Geometry: final body of the model. Coordinates: model frame, mm. A direction names the side the tool comes from. Round coordinates to 2 decimals unless told otherwise and drop trailing zeros. Order: outer loops, then holes, each group sorted by start corner. A loop starts at its lowest first (then second) coordinate and runs counter-clockwise, first axis right, second up. Notation, with made-up numbers: M -22.5,82 L 31.5,82 A29 ccw 31.5,106 Z; hole C -33.5,42 d10. An arc over 180 degrees is marked long. Put each result on its own line as item: value. Start each with the question number.
1) Material intervals for probe 1 along Z at (x, y) = (55, -3); probe 2 along X at (y, z) = (-4, 17.5); probe 3 along Y at (x, z) = (-53.5, 21), sorted ascending. Write a range as [from, to].
2) Section A-A, the plane x = -55. Return loops of the section in (y, z), then the cut area to 3 significant figures.
3) Section B-B, the plane z = 23. Return loops of the section in (x, y).
4) Section C-C, the plane y = -35. Return loops of the section in (x, z).
5) Section D-D, the plane y = -6.5. Return loops of the section in (x, z), then the cut area to 3 significant figures.
6) First-contact query: P1, Ø15, axis at y = -42.5, z = 20, coming from the -X side; P2, Ø2, axis at x = -16.5, y = -29.5, coming from the -Z side; P3, Ø1.5, axis at y = -59.5, z = 17.5, coming from the +X side; P4, Ø12, axis at x = 32, y = -71, coming from the +Z side. Flat tips, straight axial feed; report the tip coordinate or a pass-through.
7) Draft query along Y for faces 1 (the flat face through (-59, -15, 19)), 2 (the cylindrical face through (-59, -8, 12)), 3 (the cylindrical face through (1, -35, -10)). Return one class per face: pulls with the +Y half, pulls with the -Y half, needs draft (parallel to the pull), parting line crosses it, or undercut.
8) Access query for faces 4 (the flat face through (-55, -43, 0)), 5 (the flat face through (55, -43, 0)), 6 (the cylindrical face through (0, -75, 15)). Directions: +Z, -Z, +X, -X, +Y, -Y. A direction counts if a zero-diameter tool reaches every point of the face in a straight line with its end or side. Return the directions, or none.
from build123d import *

# Parameters (mm, degrees)
F0_W      = 140
F0_H      = 60
F1_DEPTH  = 70
F3_DEPTH  = 165
F4_W      = 30
F4_H      = 30
F5_DEPTH  = 55
F6_W      = 30
F6_H      = 30
F7_DEPTH  = 55
F8_R      = 5
F9_DEPTH  = 40
F10_R     = 5
F11_DEPTH = 40
F13_DEPTH = 100
F14_DEPTH = 10


with BuildPart() as f1:
    # F0 (on Front) → F1 (new body)
    with BuildSketch(Plane.XZ):
        Rectangle(F0_W, F0_H)
    extrude(amount=F1_DEPTH)

    # F2 (on face) → F3 (cut, symmetric)
    with BuildSketch(Plane.YZ.offset(70)):
        with BuildLine():
            Line((-55, -30), (-15, -30))
            ThreePointArc((-15, -30), (-35, -10), (-55, -30))
        make_face()
    extrude(amount=F3_DEPTH, both=True, mode=Mode.SUBTRACT)

    # F4 (on face) → F5 (cut)
    with BuildSketch(Plane.XZ.offset(70)):
        with Locations((55, 15)):
            Rectangle(F4_W, F4_H)
    extrude(amount=-F5_DEPTH, mode=Mode.SUBTRACT)

    # F6 (on face) → F7 (cut)
    with BuildSketch(Plane.XZ.offset(70)):
        with Locations((-55, 15)):
            Rectangle(F6_W, F6_H)
    extrude(amount=-F7_DEPTH, mode=Mode.SUBTRACT)

    # F8 (on face) → F9 (cut)
    with BuildSketch(Plane.XZ.offset(15)):
        with Locations((55, 15)):
            Circle(F8_R)
    extrude(amount=-F9_DEPTH, mode=Mode.SUBTRACT)

    # F10 (on face) → F11 (cut)
    with BuildSketch(Plane.XZ.offset(15)):
        with Locations((-55, 15)):
            Circle(F10_R)
    extrude(amount=-F11_DEPTH, mode=Mode.SUBTRACT)

    # F12 (on face) → F13 (cut)
    with BuildSketch(Plane.XZ.offset(70)):
        with BuildLine():
            ThreePointArc((-10, 30), (0, 20), (10, 30))
            Line((10, 30), (-10, 30))
        make_face()
        with BuildLine():
            Line((-10, 30), (10, 30))
            ThreePointArc((10, 30), (0, 40), (-10, 30))
        make_face()
        with BuildLine():
            ThreePointArc((-10, 30), (0, 40), (10, 30))
            Line((10, 30), (15, 30))
            ThreePointArc((15, 30), (0, 45), (-15, 30))
            Line((-15, 30), (-10, 30))
        make_face()
    extrude(amount=-F13_DEPTH, mode=Mode.SUBTRACT)

    # F12 (on face) → F14 (join)
    with BuildSketch(Plane.XZ.offset(70)):
        with BuildLine():
            Line((15, 30), (10, 30))
            ThreePointArc((10, 30), (0, 20), (-10, 30))
            Line((-10, 30), (-15, 30))
            ThreePointArc((-15, 30), (0, 15), (15, 30))
        make_face()
    extrude(amount=F14_DEPTH)


solid = f1.part
Result sheet:
1. probe 1: z = [-30, 10], [20, 30]
1. probe 2: x = [-70, -59.33], [-50.67, 50.67], [59.33, 70]
1. probe 3: y = [-15, 0]
2. outline: M -70,-30 L -55,-30 A20 cw -15,-30 L 0,-30 L 0,10 L -15,10 L -15,0 L -70,0 Z; M -15,20 L 0,20 L 0,30 L -15,30 Z
2. area: 1,770 mm2
3. outline: M -70,-15 L -40,-15 L -40,-70 L -13.27,-70 L -13.27,-80 L -7.14,-80 L -7.14,0 L -70,0 Z; M 7.14,-80 L 13.27,-80 L 13.27,-70 L 40,-70 L 40,-15 L 70,-15 L 70,0 L 7.14,0 Z
4. outline: M -70,-10 L 70,-10 L 70,0 L 40,0 L 40,30 L 10,30 A10 cw -10,30 L -40,30 L -40,0 L -70,0 Z
5. outline: M -70,-30 L 70,-30 L 70,30 L 10,30 A10 cw -10,30 L -70,30 Z; hole C -55,15 d10; hole C 55,15 d10
5. area: 8,090 mm2
6. P1: stops at x = -40
6. P2: stops at z = -11.09
6. P3: stops at x = 40
6. P4: stops at z = 30
7. face 1: pulls with the -Y half
7. face 2: needs draft
7. face 3: undercut
8. face 4: +Z, -X, -Y
8. face 5: +Z, +X, -Y
8. face 6: -Z, -Y
